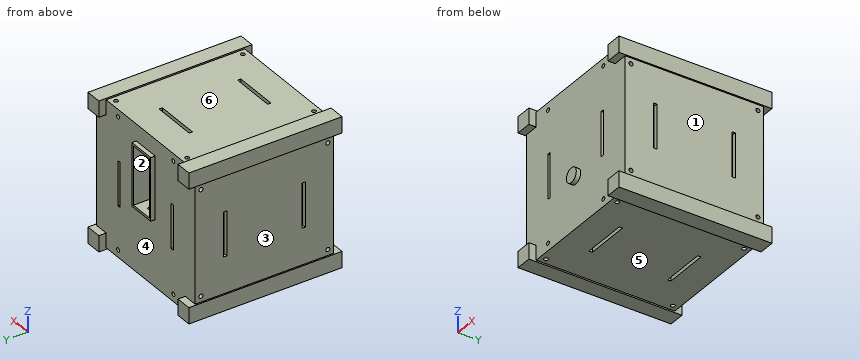
```python
from build123d import *

# Parameters (mm, degrees)
SKETCH1_W           = 100
SKETCH1_H           = 100
BOSS_EXTRUDE1_DEPTH = 95
SKETCH2_W           = 10
SKETCH2_H           = 10
BOSS_EXTRUDE2_DEPTH = 105
SKETCH3_R           = 1.4
CUT_EXTRUDE1_DEPTH  = 10
SKETCH4_W           = 11
SKETCH4_H           = 11
BOSS_EXTRUDE3_DEPTH = 105
SKETCH5_R           = 1.4
CUT_EXTRUDE2_DEPTH  = 10
SKETCH6_R           = 1.4
CUT_EXTRUDE3_DEPTH  = 10
SKETCH7_W           = 19
SKETCH7_H           = 43
SKETCH7_W_2         = 16
SKETCH7_H_2         = 40
BOSS_EXTRUDE4_DEPTH = 3
SKETCH8_W           = 16
SKETCH8_H           = 40
CUT_EXTRUDE4_DEPTH  = 10
CHAMFER2_SIZE       = 13
SKETCH9_W           = 16
SKETCH9_H           = 3.1
CUT_EXTRUDE5_DEPTH  = 10
FILLET1_R           = 1
SKETCH10_R          = 1.4
CUT_EXTRUDE6_DEPTH  = 10
SKETCH11_R          = 5
BOSS_EXTRUDE5_DEPTH = 3
SKETCH12_W          = 30.5
SKETCH12_H          = 2.2
CUT_EXTRUDE7_DEPTH  = 3
SKETCH13_W          = 30.5
SKETCH13_H          = 2.2
CUT_EXTRUDE8_DEPTH  = 3
SKETCH14_W          = 2.2
SKETCH14_H          = 30.5
CUT_EXTRUDE9_DEPTH  = 3


with BuildPart() as part:
    # Sketch1 → Boss-Extrude1 (new body)
    with BuildSketch(Plane(origin=(0, 0, 0), x_dir=(1, 0, 0), z_dir=(0, 1, 0))):
        Rectangle(SKETCH1_W, SKETCH1_H)
    extrude(amount=BOSS_EXTRUDE1_DEPTH)

    # Sketch2 → Boss-Extrude2 (add)
    with BuildSketch(Plane(origin=(0, 100, 0), x_dir=(1, 0, 0), z_dir=(0, 1, 0))):
        with Locations((-45, 45)):
            Rectangle(SKETCH2_W, SKETCH2_H)
        with Locations((45, 45)):
            Rectangle(SKETCH2_W, SKETCH2_H)
        with Locations((45, -45)):
            Rectangle(SKETCH2_W, SKETCH2_H)
        with Locations((-45, -45)):
            Rectangle(SKETCH2_W, SKETCH2_H)
    extrude(amount=-BOSS_EXTRUDE2_DEPTH)

    # Sketch3 → Cut-Extrude1 (cut)
    with BuildSketch(Plane(origin=(0, 95, 0), x_dir=(1, 0, 0), z_dir=(0, 1, 0))):
        with Locations(Location((-28, -45, 0), (0, 0, 270))):
            Circle(SKETCH3_R)
        with Locations(Location((28, -45, 0), (0, 0, 90))):
            Circle(SKETCH3_R)
        with Locations(Location((28, 45, 0), (0, 0, 270))):
            Circle(SKETCH3_R)
        with Locations(Location((-28, 45, 0), (0, 0, 90))):
            Circle(SKETCH3_R)
    cut_extrude1 = extrude(amount=-CUT_EXTRUDE1_DEPTH, mode=Mode.SUBTRACT)

    # Sketch4 → Boss-Extrude3 (add)
    with BuildSketch(Plane(origin=(0, 100, 0), x_dir=(1, 0, 0), z_dir=(0, 1, 0))):
        with Locations((-45.5, 45.5)):
            Rectangle(SKETCH4_W, SKETCH4_H)
        with Locations((45.5, 45.5)):
            Rectangle(SKETCH4_W, SKETCH4_H)
        with Locations((45.5, -45.5)):
            Rectangle(SKETCH4_W, SKETCH4_H)
        with Locations((-45.5, -45.5)):
            Rectangle(SKETCH4_W, SKETCH4_H)
    extrude(amount=-BOSS_EXTRUDE3_DEPTH)

    # Sketch5 → Cut-Extrude2 (cut)
    with BuildSketch(Plane.XY.offset(50)):
        with Locations((-36, 91)):
            Circle(SKETCH5_R)
        with Locations(Location((36, 91, 0), (0, 0, 180))):
            Circle(SKETCH5_R)
        with Locations((36, 4)):
            Circle(SKETCH5_R)
        with Locations(Location((-36, 4, 0), (0, 0, 180))):
            Circle(SKETCH5_R)
    cut_extrude2 = extrude(amount=-CUT_EXTRUDE2_DEPTH, mode=Mode.SUBTRACT)

    # Mirror1: Cut-Extrude2 across plane
    add(cut_extrude2.mirror(Plane.XY), mode=Mode.SUBTRACT)

    # Sketch6 → Cut-Extrude3 (cut)
    with BuildSketch(Plane.ZY.offset(50)):
        with Locations((-36, 91)):
            Circle(SKETCH6_R)
        with Locations(Location((36, 91, 0), (0, 0, 180))):
            Circle(SKETCH6_R)
        with Locations((36, 4)):
            Circle(SKETCH6_R)
        with Locations(Location((-36, 4, 0), (0, 0, 180))):
            Circle(SKETCH6_R)
    cut_extrude3 = extrude(amount=-CUT_EXTRUDE3_DEPTH, mode=Mode.SUBTRACT)

    # Mirror2: Cut-Extrude3 across plane
    add(cut_extrude3.mirror(Plane(origin=(0, 0, 0), x_dir=(0, 0, 1), z_dir=(1, 0, 0))), mode=Mode.SUBTRACT)

    # Mirror3: Cut-Extrude1 across plane
    add(cut_extrude1.mirror(Plane.ZX.offset(47.5)), mode=Mode.SUBTRACT)

    # Sketch7 → Boss-Extrude4 (add)
    with BuildSketch(Plane(origin=(0, 95, 0), x_dir=(1, 0, 0), z_dir=(0, 1, 0))):
        with Locations((0, -17)):
            Rectangle(SKETCH7_W, SKETCH7_H)
        with Locations((0, -17)):
            Rectangle(SKETCH7_W_2, SKETCH7_H_2, mode=Mode.SUBTRACT)
    extrude(amount=BOSS_EXTRUDE4_DEPTH)

    # Sketch8 → Cut-Extrude4 (cut)
    with BuildSketch(Plane(origin=(0, 95, 0), x_dir=(1, 0, 0), z_dir=(0, 1, 0))):
        with Locations((0, -17)):
            Rectangle(SKETCH8_W, SKETCH8_H)
    extrude(amount=-CUT_EXTRUDE4_DEPTH, mode=Mode.SUBTRACT)

    # Chamfer2
    chamfer2_edges = [part.edges().sort_by_distance(p)[0] for p in [
        (0, 85, 37),
    ]]
    chamfer(chamfer2_edges, length=CHAMFER2_SIZE - 0.0001)  # a hair under: the kernel refuses the full size

    # Sketch9 → Cut-Extrude5 (cut)
    with BuildSketch(Plane(origin=(0, 85, 0), x_dir=(1, 0, 0), z_dir=(0, 1, 0))):
        with Locations((0, 1.45)):
            Rectangle(SKETCH9_W, SKETCH9_H)
    extrude(amount=-CUT_EXTRUDE5_DEPTH, mode=Mode.SUBTRACT)

    # Fillet1
    fillet1_edges = [part.edges().sort_by_distance(p)[0] for p in [
        (0, 85, 0.1),
    ]]
    fillet(fillet1_edges, radius=FILLET1_R)

    # Sketch10 → Cut-Extrude6 (cut)
    with BuildSketch(Plane.XY.offset(-3)):
        with Locations((0, 92)):
            Circle(SKETCH10_R)
    extrude(amount=-CUT_EXTRUDE6_DEPTH, mode=Mode.SUBTRACT)

    # Sketch11 → Boss-Extrude5 (add)
    with BuildSketch(Plane.XZ):
        with Locations(Location((0, -15, 0), (0, 0, 90))):
            Circle(SKETCH11_R)
    extrude(amount=BOSS_EXTRUDE5_DEPTH)

    # Sketch12 → Cut-Extrude7 (cut)
    with BuildSketch(Plane.ZY.offset(50)):
        with Locations((0, 74.4)):
            Rectangle(SKETCH12_W, SKETCH12_H)
        with Locations((0, 20.6)):
            Rectangle(SKETCH12_W, SKETCH12_H)
    cut_extrude7 = extrude(amount=-CUT_EXTRUDE7_DEPTH, mode=Mode.SUBTRACT)

    # Mirror4: Cut-Extrude7 across plane
    add(cut_extrude7.mirror(Plane(origin=(0, 0, 0), x_dir=(0, 0, 1), z_dir=(1, 0, 0))), mode=Mode.SUBTRACT)

    # Sketch13 → Cut-Extrude8 (cut)
    with BuildSketch(Plane.XY.offset(50)):
        with Locations((0, 74.4)):
            Rectangle(SKETCH13_W, SKETCH13_H)
        with Locations((0, 20.6)):
            Rectangle(SKETCH13_W, SKETCH13_H)
    cut_extrude8 = extrude(amount=-CUT_EXTRUDE8_DEPTH, mode=Mode.SUBTRACT)

    # Mirror5: Cut-Extrude8 across plane
    add(cut_extrude8.mirror(Plane.XY), mode=Mode.SUBTRACT)

    # Sketch14 → Cut-Extrude9 (cut)
    with BuildSketch(Plane(origin=(0, 95, 0), x_dir=(1, 0, 0), z_dir=(0, 1, 0))):
        with Locations((26.9, 0)):
            Rectangle(SKETCH14_W, SKETCH14_H)
        with Locations((-26.9, 0)):
            Rectangle(SKETCH14_W, SKETCH14_H)
    cut_extrude9 = extrude(amount=-CUT_EXTRUDE9_DEPTH, mode=Mode.SUBTRACT)

    # Mirror6: Cut-Extrude9 across plane
    add(cut_extrude9.mirror(Plane.ZX.offset(47.5)), mode=Mode.SUBTRACT)


solid = part.part
```
Verification items for the finished model (mm, model axes). Face numbers are marked on the shaded views. A direction names the side the tool comes from. Coordinates: 2 decimals unless noted, no trailing zeros. Order: outer loops, then holes, each group sorted by start corner. A loop starts at its lowest first (then second) coordinate and runs counter-clockwise, first axis right, second up. Notation, with made-up numbers: (7.25, 67.5) -> (36.25, 67.5) arc R24 cw to (36.25, 96.5) -> close; hole circle Ø9 at (44.25, -10). An arc over 180 degrees is marked (long way). Answer as CSV lines item,"result". Start each with the question number.
1) Gauge pin test, flat ends, axial feed: pin 1 Ø0.9 at (x, z) = (3.5, 48) entering from -Y; pin 2 Ø5 at (x, z) = (19, -23) entering from +Y; pin 3 Ø0.8 at (x, z) = (27.5, 45.5) entering from +Y. Record the tip position at first contact, or that the pin passes through.
2) Cross-section at C-C, the plane x = -41.5. Record the boundary of the cut face in (y, z), then the cut area to 3 significant figures.
3) Cross-section at D-D, the plane x = -31. Record the boundary of the cut face in (y, z), then the cut area to 3 significant figures.
4) Set-up check for the marked faces 1 and 2: record each of +Z, -Z, +X, -X, +Y, -Y from which the full face is reachable in a straight line by a thin tool's end or side.
5) Cross-section at B-B, the plane y = 55.5. Record the boundary of the cut face in (x, z).
6) Release check for a two-part mould opening along Z. For the marked faces 3, 4, 5 and 6 record: released by +Z, released by -Z, zero draft, split by the parting line, or undercut.
7) Cross-section at A-A, the plane y = 78. Record the boundary of the cut face in (x, z), then the cut area to 3 significant figures.
8) Material ranges on L1, parallel to Y at x = -47, z = 36; L2, parallel to X at y = 94, z = -5; L3, parallel to X at y = 53, z = 9, recorded low to high. Write a range as [from, to].
Conclusion:
1,pin 1,"stops at y = 0"
1,pin 2,"stops at y = 95"
1,pin 3,"stops at y = 85"
2,outline,"(-5, -51) -> (100, -51) -> (100, -40) -> (95, -40) -> (95, 40) -> (100, 40) -> (100, 51) -> (-5, 51) -> (-5, 40) -> (0, 40) -> (0, -40) -> (-5, -40) -> close; hole circle Ø2.8 at (4, -36); hole circle Ø2.8 at (4, 36); hole circle Ø2.8 at (91, -36); hole circle Ø2.8 at (91, 36)"
2,area,"9,890 mm²"
3,outline,"(0, -50) -> (95, -50) -> (95, 50) -> (0, 50) -> close"
3,area,"9,500 mm²"
4,face 1,"+X, +Y, -Y"
4,face 2,"+Y"
5,outline,"(-51, -51) -> (-40, -51) -> (-40, -50) -> (40, -50) -> (40, -51) -> (51, -51) -> (51, -40) -> (50, -40) -> (50, 40) -> (51, 40) -> (51, 51) -> (40, 51) -> (40, 50) -> (-40, 50) -> (-40, 51) -> (-51, 51) -> (-51, 40) -> (-50, 40) -> (-50, -40) -> (-51, -40) -> close"
6,face 3,"undercut"
6,face 4,"undercut"
6,face 5,"released by -Z"
6,face 6,"released by +Z"
7,outline,"(-51, -51) -> (-40, -51) -> (-40, -50) -> (40, -50) -> (40, -51) -> (51, -51) -> (51, -40) -> (50, -40) -> (50, 40) -> (51, 40) -> (51, 51) -> (40, 51) -> (40, 50) -> (-40, 50) -> (-40, 51) -> (-51, 51) -> (-51, 40) -> (-50, 40) -> (-50, -40) -> (-51, -40) -> close; hole (-8, -3) -> (8, -3) -> (8, 0.1) -> (-8, 0.1) -> close"
7,area,"10,000 mm²"
8,L1,"y = [0, 2.6], [5.4, 89.6], [92.4, 95]"
8,L2,"x = [-50, -28], [-25.8, 25.8], [28, 50]"
8,L3,"x = [-50, 50]"
